Source: CAD feature listing. Evaluate the final solid. Frame: model axes, mm. Round coordinates to 2 decimals unless told otherwise and drop trailing zeros. Loops run counter-clockwise (first coordinate to the right, second up) from the corner with the lowest first, then second, coordinate; pieces in that order, holes last.
(1) Section A-A, the plane x = -55. Return the cut outline in (y, z), plus the area to 3 significant figures.
(2) First-contact query: pin 1 Ø6.5 at (x, y) = (-55, 15) entering from -Z; pin 2 Ø1.9 at (x, y) = (-22.5, 0) entering from +Z. Flat tips, straight axial feed; report the tip coordinate or a pass-through.
(3) Section B-B, the plane y = -15. Return the cut outline in (x, z).
(4) Material intervals for probe 1 along Y at (x, z) = (55, 0.85); probe 2 along Y at (x, z) = (-22.5, 1.6); probe 3 along X at (y, z) = (15.5, 1.45), sorted ascending.
(5) Section C-C, the plane x = 22.5. Return the cut outline in (y, z), plus the area to 3 significant figures.
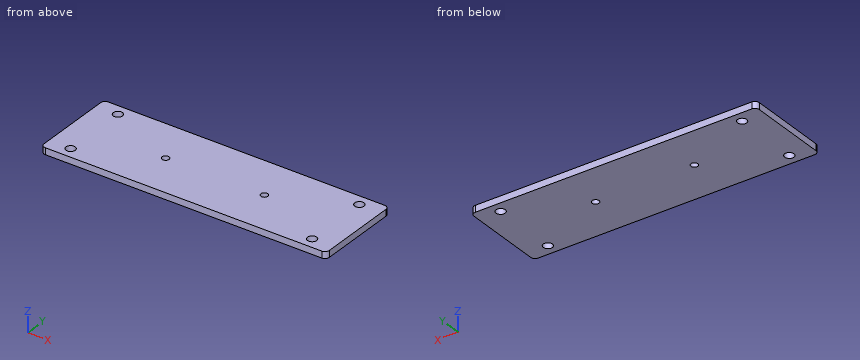
Autodesk Inventor part; units mm, degrees
ref_plane "YZ Plane" through (0, 0, 0) normal (1, 0, 0) x (0, 1, 0)
ref_plane "XZ Plane" through (0, 0, 0) normal (0, 1, 0) x (-1, 0, 0)
ref_plane "XY Plane" through (0, 0, 0) normal (0, 0, 1) x (1, 0, 0)
sketch "スケッチ1" plane through (0, 0, 0) normal (0, 0, 1) x (1, 0, 0)
  line L0 (65, -20) -> (-65, -20)
  line L1 (-65, -20) -> (-65, 20)
  line L2 (-65, 20) -> (65, 20)
  line L3 (65, 20) -> (65, -20)
  line L4 (65, -20) -> (-65, 20) construction
  line L5 (-65, -20) -> (65, 20) construction
  circle A0 centre (-55, 15) radius 2.1
  circle A1 centre (-55, -15) radius 2.1
  circle A2 centre (55, 15) radius 2.1
  circle A3 centre (55, -15) radius 2.1
  circle A4 centre (22.5, 0) radius 1.6
  circle A5 centre (-22.5, 0) radius 1.6
  point P0 (0, 0)
  point P1 (0, 0)
  dimension "d0" = 130
  dimension "d1" = 40
  dimension "d2" = 4.2
  dimension "d3" = 4.2
  dimension "d4" = 4.2
  dimension "d5" = 4.2
  dimension "d6" = 3.2
  dimension "d7" = 3.2
  dimension "d8" = 22.5
  dimension "d9" = 22.5
  dimension "d10" = 10
  dimension "d11" = 10
  dimension "d12" = 5
  dimension "d13" = 5
  dimension "d14" = 10
  dimension "d15" = 5
  dimension "d16" = 10
  dimension "d17" = 5
extrude "押し出し1" add sketch "スケッチ1" along normal blind 3
fillet "フィレット1" radius 2 4 edges at (65, 20, 1.5) (65, -20, 1.5) (-65, 20, 1.5) (-65, -20, 1.5)
properties part number "RPlate"
Output values:
1. outline: (-20, 0) - (-17.1, 0) - (-17.1, 3) - (-20, 3) - close; (-12.9, 0) - (12.9, 0) - (12.9, 3) - (-12.9, 3) - close; (17.1, 0) - (20, 0) - (20, 3) - (17.1, 3) - close
1. area: 94.8 mm2
2. pin 1: stops at z = 0
2. pin 2: passes through
3. outline: (-65, 0) - (-57.1, 0) - (-57.1, 3) - (-65, 3) - close; (-52.9, 0) - (52.9, 0) - (52.9, 3) - (-52.9, 3) - close; (57.1, 0) - (65, 0) - (65, 3) - (57.1, 3) - close
4. probe 1: y = -20 to -17.1, -12.9 to 12.9, 17.1 to 20
4. probe 2: y = -20 to -1.6, 1.6 to 20
4. probe 3: x = -65 to -57.04, -52.96 to 52.96, 57.04 to 65
5. outline: (-20, 0) - (-1.6, 0) - (-1.6, 3) - (-20, 3) - close; (1.6, 0) - (20, 0) - (20, 3) - (1.6, 3) - close
5. area: 110 mm2
